Design review of the part built by this model. Coordinates are the model's own, in mm. Face numbers are marked on the shaded views. Coordinates: 2 decimals unless noted, no trailing zeros. Loops run counter-clockwise (first coordinate to the right, second up) from the corner with the lowest first, then second, coordinate; pieces in that order, holes last. Notation, with made-up numbers: (1.5, 80) - (27.5, 80) arc R17 ccw to (27.5, 90) - close; hole circle Ø5 at (36, -24). An arc over 180 degrees is marked (long way). Use one line per item in the form item = value. Start each with the question number.
(1) Add section A-A (y = 1.55). State the section outline as (x, z) points.
(2) Add section B-B (z = 0). Count the separate pieces of the cut face and the enclosed holes in it, plus the area to 3 significant figures.
(3) Add section D-D (z = -5.5). State the section outline as (x, y) points, plus the area to 3 significant figures.
(4) Add section C-C (x = -11.5). State the section outline as (y, z) points.
(5) Clearance check with flat-ended pins moving along their axes: pin 1 Ø2 at (x, z) = (14.5, -1.5) entering from -Y; pin 2 Ø1.8 at (x, z) = (20.15, 0) entering from -Y. State where each tip first meets the part, or that it passes through.
(6) For L1, parallel to X at y = 0.9, z = 0; L2, parallel to Y at x = -11, z = 0.5; L3, parallel to Z at x = 21, y = 0.9, list the stretches that pass through material, from the lowest coordinate up.
(7) The part is to be moulded in two halves that separate along X. For the marked faces 1 and 2, say which applies: pulls with the +X half, pulls with the -X half, needs draft (parallel to the pull), parting line crosses it, or undercut.
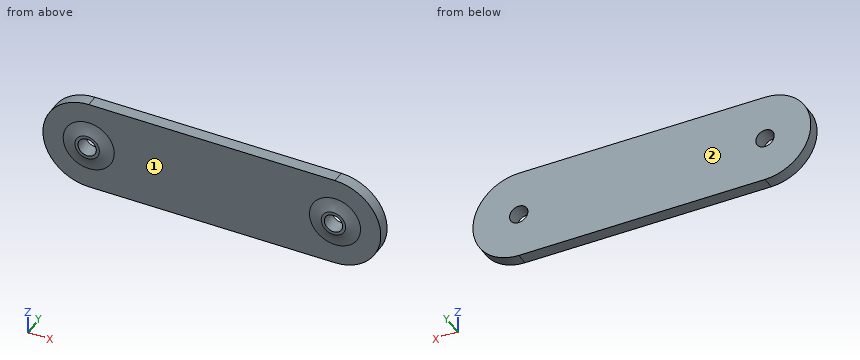
```python
from build123d import *

# Parameters (mm, degrees)
BOSS_EXTRUDE1_DEPTH = 2
SKETCH2_R           = 1.5
CUT_EXTRUDE1_DEPTH  = 29.718852693
BOSS_EXTRUDE2_START = 0.5
SKETCH3_R           = 2
SKETCH3_R_2         = 1.5
BOSS_EXTRUDE2_DEPTH = 0.5
FILLET1_R           = 5


with BuildPart() as part:
    # Sketch1 → Boss-Extrude1 (new body)
    with BuildSketch(Plane(origin=(0, 0, 0), x_dir=(1, 0, 0), z_dir=(0, 1, 0))):
        with BuildLine():
            Line((-20.15, 7.5), (20.15, 7.5))
            ThreePointArc((20.15, 7.5), (27.65, 0), (20.15, -7.5))
            Line((20.15, -7.5), (-20.15, -7.5))
            ThreePointArc((-20.15, -7.5), (-27.65, 0), (-20.15, 7.5))
        make_face()
    extrude(amount=BOSS_EXTRUDE1_DEPTH)

    # Sketch2 → Cut-Extrude1 (cut, through all)
    with BuildSketch(Plane.XZ):
        with Locations(Location((-20.15, 0, 0), (0, 0, 270))):
            Circle(SKETCH2_R)
        with Locations(Location((20.15, 0, 0), (0, 0, 270))):
            Circle(SKETCH2_R)
    extrude(amount=-CUT_EXTRUDE1_DEPTH, mode=Mode.SUBTRACT)

    # Sketch3 → Boss-Extrude2 (add)
    # profile 1 of 2: a face of its own
    with BuildSketch(Plane.XZ.offset(BOSS_EXTRUDE2_START)):
        with Locations(Location((-20.15, 0, 0), (0, 0, 90))):
            Circle(SKETCH3_R)
        with Locations(Location((-20.15, 0, 0), (0, 0, 270))):
            Circle(SKETCH3_R_2, mode=Mode.SUBTRACT)
    # profile 2 of 2: a face of its own
    with BuildSketch(Plane.XZ.offset(BOSS_EXTRUDE2_START)):
        with Locations(Location((20.15, 0, 0), (0, 0, 90))):
            Circle(SKETCH3_R)
        with Locations(Location((20.15, 0, 0), (0, 0, 270))):
            Circle(SKETCH3_R_2, mode=Mode.SUBTRACT)
    extrude(amount=-BOSS_EXTRUDE2_DEPTH)

    # Fillet1
    # the kernel refuses this fillet: 5 mm, written as the material it adds along each edge
    with BuildSketch(Plane(origin=(-20.15, 0, 0), x_dir=(0, 0, 1), z_dir=(1, 0, 0))) as fillet1_piece_1:
        with BuildLine():
            CenterArc((4.179449472, 5), FILLET1_R, 244.158067237, 25.841932763)
            Line((4.179449472, 0), (4.179449472, -0.1))
            Line((4.179449472, -0.1), (2, -0.1))
            Line((2, -0.1), (1.9, 0))
            ThreePointArc((1.9, 0), (1.9, 0.25), (1.956411011, 0.41))
            Line((1.956411011, 0.41), (2, 0.5))
        make_face()
    revolve(axis=Axis((-20.15, 0, 0), (0, -1, 0)))
    with BuildSketch(Plane(origin=(20.15, 0, 0), x_dir=(0, 0, 1), z_dir=(1, 0, 0))) as fillet1_piece_2:
        with BuildLine():
            CenterArc((4.179449472, 5), FILLET1_R, 244.158067237, 25.841932763)
            Line((4.179449472, 0), (4.179449472, -0.1))
            Line((4.179449472, -0.1), (2, -0.1))
            Line((2, -0.1), (1.9, 0))
            ThreePointArc((1.9, 0), (1.9, 0.25), (1.956411011, 0.41))
            Line((1.956411011, 0.41), (2, 0.5))
        make_face()
    revolve(axis=Axis((20.15, 0, 0), (0, -1, 0)))


solid = part.part
```
Computed values:
q1.outline = (-20.15, -7.5) - (20.15, -7.5) arc R7.5 ccw to (20.15, 7.5) - (-20.15, 7.5) arc R7.5 ccw to start; hole circle Ø3 at (-20.15, 0); hole circle Ø3 at (20.15, 0)
q2.separate_pieces = 3
q2.enclosed_holes = 0
q2.area = 101 mm^2
q3.outline = (-25.25, 0) - (25.25, 0) - (25.25, 2) - (-25.25, 2) - close
q3.area = 101 mm^2
q4.outline = (0, -7.5) - (2, -7.5) - (2, 7.5) - (0, 7.5) - close
q5.pin_1 = 0
q5.pin_2 = through
q6.L1 = -27.65 to -21.65, -18.65 to 18.65, 21.65 to 27.65
q6.L2 = 0 to 2
q6.L3 = -7.45 to -1.24, 1.24 to 7.45
q7.face_1 = undercut
q7.face_2 = needs draft
